Autodesk Inventor part; units mm, degrees
ref_plane "YZ Plane" through (0, 0, 0) normal (1, 0, 0) x (0, 1, 0)
ref_plane "XZ Plane" through (0, 0, 0) normal (0, 1, 0) x (-1, 0, 0)
ref_plane "XY Plane" through (0, 0, 0) normal (0, 0, 1) x (1, 0, 0)
sketch "Esquisse1" plane through (0, 0, 0) normal (1, 0, 0) x (0, 1, 0)
  line L0 (0, 0) -> (25, 0)
  line L1 (25, 0) -> (25, -7.347)
  line L2 (25, -7.347) -> (0, -7.347)
  line L3 (0, -7.347) -> (0, 0)
  dimension "d0" = 25
  dimension "d1" = 7.347
extrude "Extrusion1" add sketch "Esquisse1" along normal blind 10
sketch "Esquisse3" plane through (10, 0, 0) normal (1, 0, 0) x (0, 0, -1)
  line L0 (0, 0) -> (7.347, 0)
  line L1 (0, 0) -> (3.5, 0)
  line L2 (3.5, 0) -> (3.5, 4)
  line L3 (7.347, 25) -> (0, 25)
  line L4 (0, 25) -> (3.5, 25)
  line L5 (3.5, 25) -> (3.5, 21)
  dimension "d7" = 3.5
  dimension "d8" = 4
  dimension "d9" = 3.5
  dimension "d10" = 4
  dimension "d11" = 90
hole "Perçage1" at (10, 4, -3.5) at (10, 21, -3.5) direction (-1, 0, 0) diameter 1.567 end through all
sketch "Esquisse4" plane through (0, 0, 0) normal (0, 0, 1) x (1, 0, 0)
  line L0 (0, 0) -> (10, 0)
  line L1 (0, 0) -> (6.6987, 25)
  line L2 (0, 25) -> (10, 25)
  line L3 (0, 0) -> (25.8819, 0) construction
  line L4 (0, 25) -> (10, 25)
  line L5 (10, 25) -> (10, 0)
  dimension "d19" = 75
extrude "Extrusion3" cut sketch "Esquisse4" against normal blind 10
properties part number "face 15°"
Can you work these out from the model? Positions are in its coordinate system, mm. Coordinates: 2 decimals unless noted, no trailing zeros. Loops run counter-clockwise (first coordinate to the right, second up) from the corner with the lowest first, then second, coordinate; pieces in that order, holes last. Notation, with made-up numbers: (35, -28) - (88, -28) arc R22 ccw to (88, -13) - close; hole circle Ø3 at (-37.75, 44). An arc over 180 degrees is marked (long way). Answer as CSV lines item,"result". Start each with the question number.
1) Thinking about a two-plate mould opening in Y: for faces 1 (the cylindrical face through (0.49, 4.765, -3.33)), 2 (the flat face through (0, 12, -4)), 3 (the flat face through (3.302, 12.325, -3.622)), which applies, pulls with the +Y half, pulls with the -Y half, needs draft (parallel to the pull), parting line crosses it, or undercut?
2) Suppose I cut it at A-A (y = 21). Please give me the cut outline in (x, z).
3) I need wall thicknesses on line 1 (Z direction, x = 1, y = 4); line 2 (Y direction, x = 1.05, z = -3.5); line 3 (X direction, y = 18.5, z = -2.5). Which ranges of each line are inside material? Lowest first, please. Write a range as from..to.
4) Suppose I cut it at B-B (z = -3). Please give me the cut outline in (x, y), plus the area to 3 significant figures.
5) Suppose I cut it at C-C (x = 2). Please give me the cut outline in (y, z).
6) For pin 1 (1.5 mm diameter, centred on y = 8.5, z = -3.5, fed in from +X); pin 2 (2.5 mm diameter, centred on y = 4, z = -3.5, fed in from +X), each with a flat end and sliding along its axis, tell me the tip position at first contact or that it passes through.
7) Suppose I cut it at D-D (z = -7). Please give me the cut outline in (x, y).
Check result:
1,face 1,"undercut"
1,face 2,"needs draft"
1,face 3,"pulls with the -Y half"
2,outline,"(0, -7.35) - (5.63, -7.35) - (5.63, -4.28) - (0, -4.28) - close; (0, -2.72) - (5.63, -2.72) - (5.63, 0) - (0, 0) - close"
3,line 1,"z = -7.35..-4.28, -2.72..0"
3,line 2,"y = 4.78..20.22, 21.78..25"
3,line 3,"x = 0..4.96"
4,outline,"(0, 0) - (0.91, 3.4) - (0, 3.4) - close; (0, 4.6) - (1.23, 4.6) - (5.47, 20.4) - (0, 20.4) - close; (0, 21.6) - (5.79, 21.6) - (6.7, 25) - (0, 25) - close"
4,area,"75.7 mm²"
5,outline,"(7.46, -7.35) - (25, -7.35) - (25, 0) - (7.46, 0) - close; hole circle Ø1.57 at (21, -3.5)"
6,pin 1,"stops at x = 2.48"
6,pin 2,"stops at x = 1.41"
7,outline,"(0, 0) - (6.7, 25) - (0, 25) - close"
